Could you check a few things on this model? Use its own coordinates, in mm. A direction names the side the tool comes from. Give positions to 0.01 mm unless a question says otherwise; leave off trailing zeros. Order: outer loops, then holes, each group sorted by start corner. A loop starts at its lowest first (then second) coordinate and runs counter-clockwise, first axis right, second up. Notation, with made-up numbers: M 9,-37 L 64,-37 A35 ccw 64,-4 Z; hole C -20,16 d2. An arc over 180 degrees is marked long. Return JSON: item names as keys, results as strings. Group by question number.
```python
from build123d import *

# Parameters (mm, degrees)
SKETCH_1_W          = 15
SKETCH_1_H          = 15
SKETCH_1_W_2        = 13
SKETCH_1_H_2        = 13
EXTRUDE_1_DEPTH     = 400
SKETCH_2_R          = 1.45
CUT_EXTRUDE_1_DEPTH = 401.35140814
SKETCH_3_R          = 1.45
CUT_EXTRUDE_2_DEPTH = 401.35140814


with BuildPart() as part:
    # 草图1 → 凸台-拉伸1 (new body)
    with BuildSketch(Plane(origin=(0, 0, 0), x_dir=(0, 0, -1), z_dir=(1, 0, 0))):
        Rectangle(SKETCH_1_W, SKETCH_1_H)
        Rectangle(SKETCH_1_W_2, SKETCH_1_H_2, mode=Mode.SUBTRACT)
    extrude(amount=EXTRUDE_1_DEPTH)

    # 草图2 → 切除-拉伸1 (cut, through all)
    with BuildSketch(Plane.XY.offset(7.5)):
        with Locations((371, 0)):
            Circle(SKETCH_2_R)
        with Locations((361, 0)):
            Circle(SKETCH_2_R)
        with Locations((350, 0)):
            Circle(SKETCH_2_R)
        with Locations((325, 0)):
            Circle(SKETCH_2_R)
        with Locations((215, 0)):
            Circle(SKETCH_2_R)
        with Locations((200, 0)):
            Circle(SKETCH_2_R)
        with Locations((185, 0)):
            Circle(SKETCH_2_R)
        with Locations((75, 0)):
            Circle(SKETCH_2_R)
        with Locations((50, 0)):
            Circle(SKETCH_2_R)
        with Locations((39, 0)):
            Circle(SKETCH_2_R)
        with Locations((29, 0)):
            Circle(SKETCH_2_R)
    extrude(amount=-CUT_EXTRUDE_1_DEPTH, mode=Mode.SUBTRACT)

    # 草图3 → 切除-拉伸2 (cut, through all)
    with BuildSketch(Plane(origin=(0, 7.5, 0), x_dir=(1, 0, 0), z_dir=(0, 1, 0))):
        with Locations(Location((376, 0, 0), (0, 0, 270))):
            Circle(SKETCH_3_R)
        with Locations(Location((366, 0, 0), (0, 0, 270))):
            Circle(SKETCH_3_R)
        with Locations(Location((320, 0, 0), (0, 0, 270))):
            Circle(SKETCH_3_R)
        with Locations(Location((310, 0, 0), (0, 0, 270))):
            Circle(SKETCH_3_R)
        with Locations(Location((90, 0, 0), (0, 0, 270))):
            Circle(SKETCH_3_R)
        with Locations(Location((80, 0, 0), (0, 0, 270))):
            Circle(SKETCH_3_R)
        with Locations(Location((34, 0, 0), (0, 0, 270))):
            Circle(SKETCH_3_R)
        with Locations(Location((24, 0, 0), (0, 0, 270))):
            Circle(SKETCH_3_R)
    extrude(amount=-CUT_EXTRUDE_2_DEPTH, mode=Mode.SUBTRACT)


solid = part.part
```
1. Which directions (+Z, -Z, +X, -X, +Y, -Y) give clear straight access to the entire face, cutting with the end or side of a thin tool? Please do faces 4 (the flat face through (197, -6.5, 0)), 5 (the flat face through (197, 7.5, 0)).
2. I need wall thicknesses on L1, parallel to Y at x = 133, z = 0.5; L2, parallel to Z at x = 310, y = 7.3. Which ranges of each line are inside material? Lowest first, please. Write a range as from..to.
3. If we mould it in two halves opening along Z, with no side actions, what happens to faces 1 (the flat face through (197, 0, -7.5)), 2 (the flat face through (197, 6.5, 0)), 3 (the flat face through (400, 0, 7))? For each: pulls with the +Z half, pulls with the -Z half, needs draft (parallel to the pull), parting line crosses it, or undercut.
4. Imagine slicing it at B-B, the plane z = -4. Please give me the cut outline in (x, y), plus the area to 3 significant figures.
5. Imagine slicing it at A-A, the plane x = 240. Please give me the cut outline in (y, z).
Values:
{
 "1": {"face 4": "+X, -X", "face 5": "+Z, -Z, +X, -X, +Y"},
 "2": {"L1": "y = -7.5..-6.5, 6.5..7.5", "L2": "z = -7.5..-1.45, 1.45..7.5"},
 "3": {"face 1": "pulls with the -Z half", "face 2": "undercut", "face 3": "needs draft"},
 "4": {"outline": "M 0,-7.5 L 400,-7.5 L 400,-6.5 L 0,-6.5 Z; M 0,6.5 L 400,6.5 L 400,7.5 L 0,7.5 Z", "area": "800 mm²"},
 "5": {"outline": "M -7.5,-7.5 L 7.5,-7.5 L 7.5,7.5 L -7.5,7.5 Z; hole M -6.5,-6.5 L 6.5,-6.5 L 6.5,6.5 L -6.5,6.5 Z"}
}
